Build history of the part. All positions in model axes, mm. Face numbers are marked on the shaded views. A direction names the side the tool comes from. Give positions to 0.01 mm unless a question says otherwise; leave off trailing zeros. Write each loop counter-clockwise with the first axis right and the second up, starting at its lowest first coordinate (ties: lowest second). Pieces come first, ordered by that corner, then holes. Notation, with made-up numbers: (0.25, -37) - (9.25, -37) arc R20 ccw to (9.25, -24) - close; hole circle Ø7 at (35.5, -28). An arc over 180 degrees is marked (long way). Use one line per item in the form item = value. Start each with the question number.
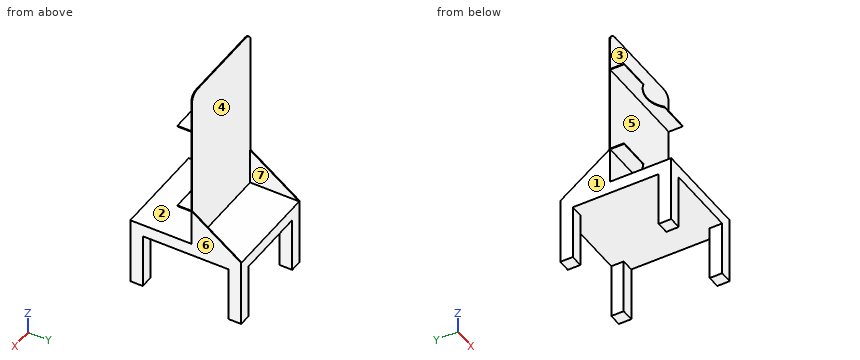
from build123d import *

# Parameters (mm, degrees)
F0_W      = 350
F0_H      = 400
F1_DEPTH  = 45
F2_W      = 45
F2_H      = 45
F3_DEPTH  = 200
F4_W      = 350
F4_H      = 3
F5_DEPTH  = 600
F6_R      = 30
F8_DEPTH  = 3
F10_DEPTH = 3
F11_W     = 350
F11_H     = 3
F12_DEPTH = 50
F14_DEPTH = 350


with BuildPart() as f1:
    # F0 (on Top) → F1 (new body)
    with BuildSketch(Plane.XY):
        Rectangle(F0_W, F0_H)
    extrude(amount=F1_DEPTH)

    # F2 (on face) → F3 (join)
    with BuildSketch(Plane(origin=(0, 0, 0), x_dir=(1, 0, 0), z_dir=(0, 0, -1))):
        with Locations((-152.5, 177.5)):
            Rectangle(F2_W, F2_H)
        with Locations((152.5, 177.5)):
            Rectangle(F2_W, F2_H)
        with Locations((-152.5, -177.5)):
            Rectangle(F2_W, F2_H)
        with Locations((152.5, -177.5)):
            Rectangle(F2_W, F2_H)
    extrude(amount=F3_DEPTH)

    # F4 (on face) → F5 (join)
    with BuildSketch(Plane.XY.offset(45)):
        with Locations((0, 21.5)):
            Rectangle(F4_W, F4_H)
    extrude(amount=F5_DEPTH)

    # F6
    f6_edges = [f1.edges().sort_by_distance(p)[0] for p in [
        (-175, 21.5, 645),
        (175, 21.5, 645),
    ]]
    fillet(f6_edges, radius=F6_R)

    # F7 (on face) → F8 (join)
    with BuildSketch(Plane.YZ.offset(175)):
        Polygon((23, 45), (200, 45), (23, 175), align=None)
    extrude(amount=-F8_DEPTH)

    # F9 (on face) → F10 (join)
    with BuildSketch(Plane(origin=(-175, 0, 0), x_dir=(0, -1, 0), z_dir=(-1, 0, 0))):
        Polygon((-23, 175), (-200, 45), (-23, 45), align=None)
    extrude(amount=-F10_DEPTH)

    # F11 (on face) → F12 (join)
    with BuildSketch(Plane.XZ.offset(-20)):
        with Locations((0, 176.5)):
            Rectangle(F11_W, F11_H)
        with Locations((0, 496.5)):
            Rectangle(F11_W, F11_H)
    extrude(amount=F12_DEPTH)

    # F13 (on face) → F14 (cut)
    with BuildSketch(Plane.XY.offset(498)):
        with BuildLine():
            ThreePointArc((-60.1428805791, -30), (-34.1496519515, -186.9669059898), (99.0832823142, -100))
            ThreePointArc((99.0832823142, -100), (91.050188304, -61.7670657343), (68.3094452076, -30))
            Line((68.3094452076, -30), (-60.1428805791, -30))
        make_face()
        with BuildLine():
            Line((-60.1428805791, -30), (68.3094452076, -30))
            ThreePointArc((68.3094452076, -30), (4.0832823142, -5), (-60.1428805791, -30))
        make_face()
    extrude(amount=-F14_DEPTH, mode=Mode.SUBTRACT)


solid = f1.part
(1) Which spindle directions (+Z, -Z, +X, -X, +Y, -Y) get a long thin tool onto all of the face, cutting with end or side? Do the marked faces 1, 2, 3 and 4. Say none if no direction does.
(2) Cut at B-B, the plane y = 170. Give the cut face in (x, z), then the cut area to 3 significant figures.
(3) Wall check: line 1 (Z direction, x = 33, y = 11.5); line 2 (Z direction, x = 58.5, y = 68); line 3 (X direction, y = 55.5, z = 108.5). Give the ranges that are in metal, low to high. Write a range as from..to.
(4) Cut at A-A, the plane z = -70. Give the cut face in (x, y), then the cut area to 3 significant figures.
(5) Cut at C-C, the plane z = 153.5. Give the cut face in (x, y).
(6) Two-plate mould, pull along X, no slides. Class the marked faces 5, 6 and 7: +X half, -X half, draft (parallel to the pull), parting line (faces both ways), or undercut.
(7) Cut at D-D, the plane x = -41. Give the cut face in (y, z), then the cut area to 3 significant figures.
(8) Pin check, flat tips, straight feed: pin 1 Ø1 at (x, y) = (12.5, 44.5) entering from +Z; pin 2 Ø15 at (x, y) = (-61.5, 3.5) entering from +Z; pin 3 Ø15 at (x, y) = (80.5, -16) entering from -Z. Stop position of each tip, or through.
Solution:
q1.face_1 = +Z, -Z, -X, +Y, -Y
q1.face_2 = +X, -X, -Y
q1.face_3 = +Z, +X, -X, -Y
q1.face_4 = +Z, +Y
q2.outline = (-175, -200) - (-130, -200) - (-130, 0) - (130, 0) - (130, -200) - (175, -200) - (175, 67.03) - (172, 67.03) - (172, 45) - (-172, 45) - (-172, 67.03) - (-175, 67.03) - close
q2.area = 33,900 mm2
q3.line_1 = 0..45, 175..178, 495..498
q3.line_2 = 0..45
q3.line_3 = -175..-172, 172..175
q4.outline = (-175, -200) - (-130, -200) - (-130, -155) - (-175, -155) - close; (-175, 155) - (-130, 155) - (-130, 200) - (-175, 200) - close; (130, -200) - (175, -200) - (175, -155) - (130, -155) - close; (130, 155) - (175, 155) - (175, 200) - (130, 200) - close
q4.area = 8,100 mm2
q5.outline = (-175, 20) - (175, 20) - (175, 52.27) - (172, 52.27) - (172, 23) - (-172, 23) - (-172, 52.27) - (-175, 52.27) - close
q6.face_5 = draft
q6.face_6 = +X half
q6.face_7 = undercut
q7.outline = (-200, 0) - (200, 0) - (200, 45) - (23, 45) - (23, 645) - (20, 645) - (20, 498) - (-16.38, 498) - (-16.38, 495) - (20, 495) - (20, 178) - (-16.38, 178) - (-16.38, 175) - (20, 175) - (20, 45) - (-200, 45) - close
q7.area = 20,000 mm2
q8.pin_1 = 45
q8.pin_2 = 498
q8.pin_3 = 0
